Geometry check sheet. Reference: the model listing, model coordinates, mm. A direction names the side the tool comes from. Give positions to 0.01 mm unless a question says otherwise; leave off trailing zeros. Write each loop counter-clockwise with the first axis right and the second up, starting at its lowest first coordinate (ties: lowest second). Pieces come first, ordered by that corner, then holes. Notation, with made-up numbers: M 37,25 L 61,25 A22 ccw 61,49 Z; hole C 70,43 d8. An arc over 180 degrees is marked long. One line per item, written item: value. Start each with the question number.
1. Cross-section at B-B on x = -24. Record the cut outline in (y, z), then the cut area to 3 significant figures.
2. Scan lines: line 1 (Z direction, x = -16.5, y = -3.5); line 2 (Y direction, x = -10.5, z = -43.5). Record each from-to range of solid material in increasing order.
3. Release check for a two-part mould opening along Z. For faces 1 (the face through (-29, 6, 0)), 2 (the face through (-29.294, 4.667, 1.265)), 3 (the face through (-12, 0, -20)) record: pulls with the +Z half, pulls with the -Z half, needs draft (parallel to the pull), parting line crosses it, or undercut.
4. Gauge pin test, flat ends, axial feed: pin 1 (15 mm diameter, centred on x = -16.5, z = -31.5, fed in from +Y); pin 2 (0.6 mm diameter, centred on x = -28, y = 5.5, fed in from -Z); pin 3 (2.5 mm diameter, centred on x = -3, y = 2.5, fed in from +Z). Record the tip position at first contact, or that the pin passes through.
5. Cross-section at A-A on z = -45. Record the cut outline in (x, y), then the cut area to 3 significant figures.
6. Cross-section at D-D on z = -12. Record the cut outline in (x, y).
7. Tool access check on faces 4 (the face through (-25, 4.826, -25)), 5 (the face through (-3, 2, -8.382)), 6 (the face through (-29, -1, 0)), 7 (the face through (0, -1, -29)), 8 (the face through (0, 6, -29)). Record the directions out of +Z, -Z, +X, -X, +Y, -Y that give a thin tool (end or side, any length) a straight path to the whole face; none if there is none.
8. Cross-section at C-C on y = -10.25. Record the cut outline in (x, z).
Autodesk Inventor part; units mm, degrees
ref_plane "YZ Plane" through (0, 0, 0) normal (1, 0, 0) x (0, 1, 0)
ref_plane "XZ Plane" through (0, 0, 0) normal (0, 1, 0) x (-1, 0, 0)
ref_plane "XY Plane" through (0, 0, 0) normal (0, 0, 1) x (1, 0, 0)
sketch "Sketch1" plane through (0, 0, 0) normal (0, 1, 0) x (-1, 0, 0)
  line L0 (0, 0) -> (50.8, 0)
  line L1 (50.8, 0) -> (50.8, -50.8)
  line L2 (50.8, -50.8) -> (0, -50.8)
  line L3 (0, -50.8) -> (0, 0)
  dimension "d0" = 50.8
  dimension "d1" = 50.8
extrude "Extrusion1" add sketch "Sketch1" along normal blind 4.826
sketch "Sketch2" plane through (0, 4.826, 0) normal (0, 1, 0) x (1, 0, 0)
  line L0 (0, 0) -> (-8.382, 0)
  line L1 (-8.382, 0) -> (-8.382, 8.382)
  line L2 (-8.382, 8.382) -> (0, 8.382)
  line L3 (0, 8.382) -> (0, 0)
  line L4 (-8.382, 8.382) -> (-50.8, 8.382)
  line L5 (-50.8, 50.8) -> (-50.8, 0)
  line L6 (-8.382, 8.382) -> (-8.382, 50.8)
  dimension "d4" = 8.382
  dimension "d5" = 8.382
extrude "Extrusion2" cut sketch "Sketch2" against normal blind 4.826
sketch "Sketch3" plane through (-8.382, 4.826, 0) normal (1, 0, 0) x (0, 0, -1)
  line L0 (0, -4.826) -> (0, 0)
  line L1 (0, 0) -> (0, 2.032)
  line L2 (0, -4.826) -> (0, -6.858)
  line L3 (0, -6.858) -> (-6.204, 3.8876)
  line L4 (0, 2.032) -> (-4.5461, -5.842)
  line L5 (0, 2.032) -> (9.0921, 2.032) construction
  point P0 (-2.5663, -2.413)
  dimension "d8" = 2.032
  dimension "d9" = 2.032
  dimension "d10" = 30
  dimension "d11" = 120
extrude "Extrusion3" add sketch "Sketch3" against normal blind 42.418
sketch "Sketch4" plane through (-8.382, 4.826, -8.382) normal (0, 0, 1) x (1, 0, 0)
  line L0 (8.382, 0) -> (8.382, 2.032)
  line L1 (8.382, 0) -> (10.414, 0) construction
  line L2 (8.382, -4.826) -> (8.382, -6.858)
  line L3 (8.382, -6.858) -> (14.7819, 4.2269)
  line L4 (8.382, 2.032) -> (14.3676, -8.3353)
  line L5 (8.382, 2.032) -> (20.3531, 2.032) construction
  line L6 (8.382, 0) -> (-42.418, 0)
  line L7 (8.382, 0) -> (8.382, -4.826)
  point P0 (10.9483, -2.413)
  dimension "d14" = 2.032
  dimension "d15" = 90
  dimension "d16" = 2.032
  dimension "d17" = 30
  dimension "d18" = 60
extrude "Extrusion4" add sketch "Sketch4" against normal blind 42.418
sketch "Sketch6" plane through (0, 0, 0) normal (0, -1, 0) x (1, 0, 0)
  line L0 (-50.8, -50.8) -> (-50.8, 0)
  line L1 (-50.8, -50.8) -> (-12.7, -50.8)
  line L2 (-12.7, -50.8) -> (-12.7, -12.7)
  line L3 (-12.7, -12.7) -> (-50.8, -12.7)
  line L4 (-50.8, -12.7) -> (-50.8, -50.8)
  point P0 (0, 0)
  dimension "d21" = 38.1
  dimension "d22" = 38.1
extrude "Extrusion5" add sketch "Sketch6" along normal blind 16.764
properties part number "corner support"
Report:
1. outline: M -16.76,-50.8 L 4.83,-50.8 L 4.83,0 L 6.86,0 L 2.41,2.57 L -2.03,0 L 0,0 L 0,-12.7 L -16.76,-12.7 Z
1. area: 895 mm^2
2. line 1: z = -50.8 to -12.7
2. line 2: y = 0 to 4.83
3. face 1: pulls with the -Z half
3. face 2: pulls with the +Z half
3. face 3: undercut
4. pin 1: stops at y = 4.83
4. pin 2: stops at z = 0
4. pin 3: stops at z = -8.38
5. outline: M -50.8,-16.76 L -12.7,-16.76 L -12.7,0 L 0,0 L 0,-2.03 L 2.57,2.41 L 0,6.86 L 0,4.83 L -50.8,4.83 Z
5. area: 895 mm^2
6. outline: M -50.8,0 L 0,0 L 0,-2.03 L 2.57,2.41 L 0,6.86 L 0,4.83 L -50.8,4.83 Z
7. face 4: -Z, -X, +Y
7. face 5: +Z, +X, +Y, -Y
7. face 6: +X, -X, -Y
7. face 7: +Z, -Z, -Y
7. face 8: +Z, -Z, -X, +Y
8. outline: M -50.8,-50.8 L -12.7,-50.8 L -12.7,-12.7 L -50.8,-12.7 Z
